Verification items for the finished model (mm, model axes). A direction names the side the tool comes from. Round coordinates to 2 decimals unless told otherwise and drop trailing zeros. Write each loop counter-clockwise with the first axis right and the second up, starting at its lowest first coordinate (ties: lowest second). Pieces come first, ordered by that corner, then holes. Notation, with made-up numbers: (-20, -15.75) - (-10, -15.75) arc R21 cw to (-10, 13.25) - close; hole circle Ø6 at (-12, -27.75). An arc over 180 degrees is marked (long way). Answer as a JSON object with one key per item and string values. Group by question number.
1) Section check C-C (z = -4.5). Enter the section's corners in (x, y) (3 decimals), then the cut area to 3 significant figures.
2) Set-up check for faces 4 (the flat face through (-6, -2, 6.5)), 5 (the flat face through (-7.375, -2, 0)), 6 (the flat face through (6, -2, -6.5)), 7 (the flat face through (-6, -2, 5.8)): record each of +Z, -Z, +X, -X, +Y, -Y from which the full face is reachable in a straight line by a thin tool's end or side.
3) Thickness scan on line 1 (Y direction, x = 7, z = 6.75). Record the ranges inside material, lowest first.
4) Section check B-B (x = 1). Enter the section's corners in (y, z) (3 decimals).
5) Mould release check, pull along Z, two halves, no side actions. Record for faces 1 (the flat face through (-6, -2, -6.5)), 2 (the flat face through (-8.075, -2, 0)), 3 (the flat face through (-6, -2, -5.8)): +Z half, -Z half, draft (parallel to the pull), parting line (faces both ways), or undercut.
6) Go/stop test with flat-tipped pins: pin 1 Ø0.5 at (x, y) = (6, -2) entering from +Z; pin 2 Ø1.1 at (x, y) = (-6, -2.5) entering from -Z; pin 3 Ø0.6 at (x, y) = (-7.5, -2) entering from +Z. Record where each tip stops, or that it passes through.
7) Section check A-A (y = -1.25). Enter the section's corners in (x, z) (3 decimals), then the cut area to 3 significant figures.
Autodesk Fusion 360 part; units mm, degrees
sketch "Sketch1" plane through (0, 0, 0) normal (0, 1, 0) x (1, 0, 0)
  line L0 (9.375, -7.575) -> (-9.375, -7.575)
  line L1 (-9.375, -7.575) -> (-9.375, 7.575)
  line L2 (-9.375, 7.575) -> (9.375, 7.575)
  line L3 (9.375, 7.575) -> (9.375, -7.575)
  line L4 (9.375, -7.575) -> (-9.375, 7.575) construction
  line L5 (-9.375, -7.575) -> (9.375, 7.575) construction
  dimension "d1" = 15.15
  dimension "d2" = 18.75
extrude "Extrude1" add sketch "Sketch1" along normal blind 15.24
fillet "Fillet1" radius 0.2 4 edges at (9.375, 7.62, 7.575) (-9.375, 7.62, 7.575) (-9.375, 7.62, -7.575) (9.375, 7.62, -7.575) 1 faces at (3.125, 15.24, 2.525)
sketch "Sketch2" plane through (0, 0, 0) normal (0, -1, 0) x (1, 0, 0)
  arc A0 (-9.375, -7.375) -> (-9.175, -7.575) centre (-9.175, -7.375) ccw
  line L0 (-9.175, -7.575) -> (9.175, -7.575)
  arc A1 (9.175, -7.575) -> (9.375, -7.375) centre (9.175, -7.375) ccw
  line L1 (9.375, -7.375) -> (9.375, 7.375)
  arc A2 (9.375, 7.375) -> (9.175, 7.575) centre (9.175, 7.375) ccw
  line L2 (9.175, 7.575) -> (-9.175, 7.575)
  arc A3 (-9.175, 7.575) -> (-9.375, 7.375) centre (-9.175, 7.375) ccw
  line L3 (-9.375, 7.375) -> (-9.375, -7.375)
  line L4 (6.5, -6.5) -> (-6.5, -6.5) construction
  line L5 (-6.5, -6.5) -> (-6.5, 6.5) construction
  line L6 (-6.5, 6.5) -> (6.5, 6.5) construction
  line L7 (6.5, 6.5) -> (6.5, -6.5) construction
  line L8 (6.5, -6.5) -> (-6.5, 6.5) construction
  line L9 (-6.5, -6.5) -> (6.5, 6.5) construction
  line L10 (-6.5, 6.5) -> (-5.5, 6.5)
  line L11 (-5.5, 6.5) -> (-5.5, 5.8)
  line L12 (-5.5, 5.8) -> (-6.5, 5.8)
  line L13 (-6.5, 5.8) -> (-6.5, 6.5)
  line L14 (6.5, 5.8) -> (5.5, 5.8)
  line L15 (5.5, 6.5) -> (6.5, 6.5)
  line L16 (5.5, 5.8) -> (5.5, 6.5)
  line L17 (6.5, 6.5) -> (6.5, 5.8)
  line L18 (-5.5, -6.5) -> (-6.5, -6.5)
  line L19 (-6.5, -5.8) -> (-5.5, -5.8)
  line L20 (-6.5, -6.5) -> (-6.5, -5.8)
  line L21 (-5.5, -5.8) -> (-5.5, -6.5)
  line L22 (6.5, -6.5) -> (5.5, -6.5)
  line L23 (5.5, -5.8) -> (6.5, -5.8)
  line L24 (5.5, -6.5) -> (5.5, -5.8)
  line L25 (6.5, -5.8) -> (6.5, -6.5)
  dimension "d7" = 13
  dimension "d8" = 13
  dimension "d9" = 1
  dimension "d10" = 0.7
  dimension "d13" = 12
  dimension "d14" = -12.3
extrude "Extrude2" add sketch "Sketch2" along normal blind 4 contours L10 L11 L12 L13 | L14 L15 L16 L17 | L18 L19 L20 L21 | L22 L23 L24 L25
chamfer "Chamfer1" distance 0.2 angle 45 8 edges at (5.5, -4, 6.15) (6, -4, 6.5) (6.5, -4, 6.15) (6, -4, 5.8) (6, -4, -5.8) (6.5, -4, -6.15) (6, -4, -6.5) (5.5, -4, -6.15) 2 faces at (-6.1667, -4, 6.2667) (-5.8333, -4, -6.2667)
sketch "Sketch3" plane through (0, 0, 0) normal (0, -1, 0) x (1, 0, 0)
  line L0 (6.5, -5.8) -> (6.5, -6.5)
  line L1 (6.5, -6.5) -> (5.5, -6.5)
  line L2 (5.5, -6.5) -> (5.5, -5.8)
  line L3 (5.5, -5.8) -> (6.5, -5.8)
  line L4 (-6.5, 5.8) -> (-6.5, 6.5)
  line L5 (-6.5, 6.5) -> (-5.5, 6.5)
  line L6 (-5.5, 6.5) -> (-5.5, 5.8)
  line L7 (-5.5, 5.8) -> (-6.5, 5.8)
  line L8 (-5.5, -5.8) -> (-5.5, -6.5)
  line L9 (-5.5, -6.5) -> (-6.5, -6.5)
  line L10 (-6.5, -6.5) -> (-6.5, -5.8)
  line L11 (-6.5, -5.8) -> (-5.5, -5.8)
  line L12 (6.5, 6.5) -> (6.5, 5.8)
  line L13 (6.5, 5.8) -> (5.5, 5.8)
  line L14 (5.5, 5.8) -> (5.5, 6.5)
  line L15 (5.5, 6.5) -> (6.5, 6.5)
  arc A0 (-9.375, -7.375) -> (-9.175, -7.575) centre (-9.175, -7.375) ccw
  line L16 (-9.175, -7.575) -> (9.175, -7.575)
  arc A1 (9.175, -7.575) -> (9.375, -7.375) centre (9.175, -7.375) ccw
  line L17 (9.375, -7.375) -> (9.375, 7.375)
  arc A2 (9.375, 7.375) -> (9.175, 7.575) centre (9.175, 7.375) ccw
  line L18 (9.175, 7.575) -> (-9.175, 7.575)
  arc A3 (-9.175, 7.575) -> (-9.375, 7.375) centre (-9.175, 7.375) ccw
  line L19 (-9.375, 7.375) -> (-9.375, -7.375)
  line L20 (0, 0) -> (-9.375, 0) construction
  line L21 (-7.375, -0.5) -> (-8.075, -0.5)
  line L22 (-8.075, -0.5) -> (-8.075, 0.5)
  line L23 (-8.075, 0.5) -> (-7.375, 0.5)
  line L24 (-7.375, 0.5) -> (-7.375, -0.5)
  line L25 (-7.375, -0.5) -> (-8.075, 0.5) construction
  line L26 (-8.075, -0.5) -> (-7.375, 0.5) construction
  point P0 (-7.725, 0)
  dimension "d20" = 0.7
  dimension "d21" = 1
extrude "Extrude3" add sketch "Sketch3" along normal blind 4 contours L21 L22 L23 L24
chamfer "Chamfer2" distance 0.2 angle 45 4 edges at (-7.725, -4, -0.5) (-8.075, -4, 0) (-7.725, -4, 0.5) (-7.375, -4, 0)
sketch "Sketch4" plane through (0, 0, 0) normal (0, -1, 0) x (1, 0, 0)
  line L0 (-7.375, 0.5) -> (-7.375, -0.5)
  line L1 (-7.375, -0.5) -> (-8.075, -0.5)
  line L2 (-8.075, -0.5) -> (-8.075, 0.5)
  line L3 (-8.075, 0.5) -> (-7.375, 0.5)
  line L4 (6.5, -5.8) -> (6.5, -6.5)
  line L5 (6.5, -6.5) -> (5.5, -6.5)
  line L6 (5.5, -6.5) -> (5.5, -5.8)
  line L7 (5.5, -5.8) -> (6.5, -5.8)
  line L8 (-6.5, 5.8) -> (-6.5, 6.5)
  line L9 (-6.5, 6.5) -> (-5.5, 6.5)
  line L10 (-5.5, 6.5) -> (-5.5, 5.8)
  line L11 (-5.5, 5.8) -> (-6.5, 5.8)
  line L12 (-5.5, -5.8) -> (-5.5, -6.5)
  line L13 (-5.5, -6.5) -> (-6.5, -6.5)
  line L14 (-6.5, -6.5) -> (-6.5, -5.8)
  line L15 (-6.5, -5.8) -> (-5.5, -5.8)
  line L16 (6.5, 6.5) -> (6.5, 5.8)
  line L17 (6.5, 5.8) -> (5.5, 5.8)
  line L18 (5.5, 5.8) -> (5.5, 6.5)
  line L19 (5.5, 6.5) -> (6.5, 6.5)
  arc A0 (-9.375, -7.375) -> (-9.175, -7.575) centre (-9.175, -7.375) ccw
  line L20 (-9.175, -7.575) -> (9.175, -7.575)
  arc A1 (9.175, -7.575) -> (9.375, -7.375) centre (9.175, -7.375) ccw
  line L21 (9.375, -7.375) -> (9.375, 7.375)
  arc A2 (9.375, 7.375) -> (9.175, 7.575) centre (9.175, 7.375) ccw
  line L22 (9.175, 7.575) -> (-9.175, 7.575)
  arc A3 (-9.175, 7.575) -> (-9.375, 7.375) centre (-9.175, 7.375) ccw
  line L23 (-9.375, 7.375) -> (-9.375, -7.375)
  circle A4 centre (-6, 0) radius 0.75
  dimension "d25" = 1.5
extrude "Extrude4" cut sketch "Sketch4" against normal blind 0.1 contours A4
sketch "Sketch5" plane through (0, 0.1, 0) normal (0, -1, 0) x (1, 0, 0)
  circle A0 centre (-6, 0) radius 0.75
  circle A1 centre (-6, 0) radius 0.1
extrude "Extrude5" add sketch "Sketch5" along normal blind 0.1 contours A1
sketch "Sketch6" plane through (0, 15.24, 0) normal (0, 1, 0) x (-1, 0, 0)
  line L0 (-9.175, -7.375) -> (9.175, -7.375)
  line L1 (9.175, -7.375) -> (9.175, 7.375)
  line L2 (9.175, 7.375) -> (-9.175, 7.375)
  line L3 (-9.175, 7.375) -> (-9.175, -7.375)
  line L4 (8.7536, 0.8698) -> (9.5964, 0.8698)
  line L5 (9.5964, 0.8698) -> (9.5964, -0.8698)
  line L6 (9.5964, -0.8698) -> (8.7536, -0.8698)
  line L7 (8.7536, -0.8698) -> (8.7536, 0.8698)
  line L8 (8.7536, 0.8698) -> (9.5964, -0.8698) construction
  line L9 (9.5964, 0.8698) -> (8.7536, -0.8698) construction
  circle A0 centre (8.8509, 7.0451) radius 0.2772
  point P0 (9.175, 0)
extrude "Extrude6" cut sketch "Sketch6" against normal blind 0.1 contours L1 L4 L6 L7 | L1 L4 L5 L6 | A0
Returned:
{
 "1": {"outline": "(-9.375, 0) - (9.375, 0) - (9.375, 15.04) arc R0.2 ccw to (9.175, 15.24) - (-9.175, 15.24) arc R0.2 ccw to (-9.375, 15.04) - close", "area": "286 mm2"},
 "2": {"face 4": "+Z, +X, -X, -Y", "face 5": "+Z, -Z, +X, -Y", "face 6": "-Z, +X, -X, -Y", "face 7": "+X, -X, -Y"},
 "3": {"line 1": "0 to 15.24"},
 "4": {"outline": "(0, -7.575) - (15.04, -7.575) arc R0.2 ccw to (15.24, -7.375) - (15.24, 7.375) arc R0.2 ccw to (15.04, 7.575) - (0, 7.575) - close"},
 "5": {"face 1": "-Z half", "face 2": "draft", "face 3": "undercut"},
 "6": {"pin 1": "z = 6.5", "pin 2": "z = -6.5", "pin 3": "z = 0.5"},
 "7": {"outline": "(-8.075, -0.5) - (-7.375, -0.5) - (-7.375, 0.5) - (-8.075, 0.5) - close; (-6.5, -6.5) - (-5.5, -6.5) - (-5.5, -5.8) - (-6.5, -5.8) - close; (-6.5, 5.8) - (-5.5, 5.8) - (-5.5, 6.5) - (-6.5, 6.5) - close; (5.5, -6.5) - (6.5, -6.5) - (6.5, -5.8) - (5.5, -5.8) - close; (5.5, 5.8) - (6.5, 5.8) - (6.5, 6.5) - (5.5, 6.5) - close", "area": "3.50 mm2"}
}
